For this review, take the finished solid that the model builds, in its own axes (mm). A direction names the side the tool comes from. Round coordinates to 2 decimals unless told otherwise and drop trailing zeros. Write each loop counter-clockwise with the first axis right and the second up, starting at its lowest first coordinate (ties: lowest second). Pieces come first, ordered by that corner, then holes. Notation, with made-up numbers: (79.25, -19) - (115.25, -19) arc R7 ccw to (115.25, -7) - close; hole circle Ø9 at (15.25, 24). An arc over 180 degrees is marked (long way). One line per item, written item: value. Start each with the question number.
Q1. Clearance check with flat-ended pins moving along their axes: pin 1 Ø6 at (x, z) = (13.5, 77) entering from -Y; pin 2 Ø2 at (x, y) = (-6.5, 28) entering from +Z; pin 3 Ø7.5 at (y, z) = (-4, 79.5) entering from +X. State where each tip first meets the part, or that it passes through.
Q2. Add section A-A on z = 42.5. Write out the cut boundary in (x, y).
Q3. Mouldability with a two-part tool opening along X and no side actions: class faces 4 (the face through (12.5, 0, 83)), 5 (the face through (0, 0, 45)), 6 (the face through (-37.5, 1, 35)) as +X half, -X half, draft (parallel to the pull), parting line (faces both ways), or undercut.
Q4. For probe 1 along X at (y, z) = (9, 34); probe 2 along Z at (x, y) = (12, 3); probe 3 along X at (y, z) = (-28.5, 58.5), list the stretches that pass through material, from the lowest coordinate up.
Q5. Tool access review of faces 1 (the face through (20, 20, 77)), 2 (the face through (2, -18, 20)), 3 (the face through (-12.5, -20, 15)): name each direction out of +Z, -Z, +X, -X, +Y, -Y from which nothing blocks a thin tool from reaching the whole face with its end or side.
```python
from build123d import *

# Parameters (mm, degrees)
F5_W           = 75
F5_H           = 75
F4_W           = 25
F4_H           = 25
F7_W           = 25
F7_H           = 25
F10_DEPTH      = 70.0000001
F11_DEPTH      = 70.00000015
F12_DEPTH      = 70.00000015
F14_DEPTH      = 37.5
F14_DEPTH_BACK = 12.5
F16_REACH      = 107.0166212872
F18_DEPTH      = 25


with BuildPart() as f6:
    # F5 (on offset) → F6 section 0
    with BuildSketch(Plane.XY.offset(70)):
        Rectangle(F5_W, F5_H)
    # F4 (on offset) → F6 section 1
    with BuildSketch(Plane.XY.offset(95)):
        Rectangle(F4_W, F4_H)
    loft()

    # F5 (on offset) → F8 section 0
    with BuildSketch(Plane.XY.offset(70)):
        Rectangle(F5_W, F5_H)
    # F7 (on offset) → F8 section 1
    with BuildSketch(Plane.XY.offset(45)):
        Rectangle(F7_W, F7_H)
    loft()

    # F9 (on Top) → F10 (join, through all)
    with BuildSketch(Plane.XY):
        Polygon((37.5, 37.5), (-37.5, 37.5), (-12.5, 12.5), (12.5, 12.5), align=None)
    extrude(amount=F10_DEPTH)

    # F9 (on Top) → F11 (join, through all)
    with BuildSketch(Plane.XY):
        Polygon((-37.5, 37.5), (-37.5, -37.5), (-12.5, -12.5), (-12.5, 12.5), align=None)
    extrude(amount=F11_DEPTH)

    # F9 (on Top) → F12 (join, through all)
    with BuildSketch(Plane.XY):
        Polygon((12.5, -12.5), (37.5, -37.5), (37.5, 37.5), (12.5, 12.5), align=None)
    extrude(amount=F12_DEPTH)

    # F13 (on Right) → F14 (join, two sides)
    with BuildSketch(Plane.YZ) as f14_sk:
        Polygon((-37.5, 20), (-12.5, 0), (12.5, 0), (12.5, 20), align=None)
    extrude(amount=F14_DEPTH)
    extrude(f14_sk.sketch, amount=-F14_DEPTH_BACK)

    f16_end = f6.faces().sort_by_distance((-25.9057971014, -25.9057971014, 29.2028985507))[0]
    # F15 (on face) → F16 (cut, up to a face of the model that its end follows)
    with BuildSketch(Plane.YZ.offset(37.5)):
        Polygon((-37.5, 0), (-12.5, 0), (-37.5, 20), align=None)
    f16_long = extrude(amount=-F16_REACH, mode=Mode.PRIVATE)
    add(split(f16_long, bisect_by=f16_end, keep=Keep.TOP, mode=Mode.PRIVATE), mode=Mode.SUBTRACT)

    # F17 (on offset) → F18 (cut, through all)
    with BuildSketch(Plane.XY.offset(95)):
        Polygon((12.5, 12.5), (12.5, -12.5), (37.5, -37.5), (37.5, -12.5), (37.5, 37.5), align=None)
    extrude(amount=-F18_DEPTH, mode=Mode.SUBTRACT)


solid = f6.part
```
Result set:
1. pin 1: stops at y = -33.5
1. pin 2: stops at z = 80.5
1. pin 3: stops at x = 12.5
2. outline: (-37.5, -37.5) - (-12.5, -12.5) - (-12.5, 12.5) - (12.5, 12.5) - (12.5, -12.5) - (37.5, -37.5) - (37.5, 37.5) - (-37.5, 37.5) - close
3. face 4: +X half
3. face 5: undercut
3. face 6: -X half
4. probe 1: x = -37.5 to -12.5, 12.5 to 37.5
4. probe 2: z = 0 to 20, 45 to 95
4. probe 3: x = -37.5 to -28.5, 28.5 to 37.5
5. face 1: +Z, +X
5. face 2: -Y
5. face 3: -Z, -Y
